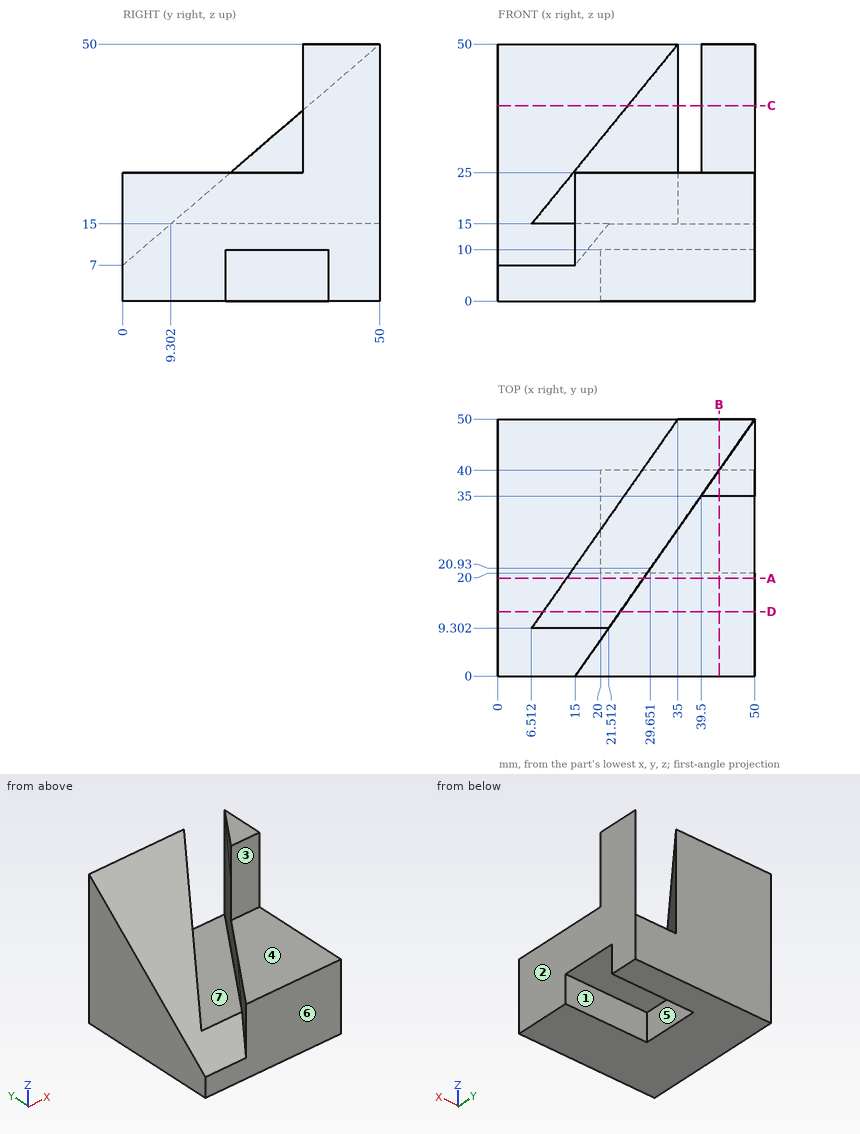
Can you work these out from the drawing? Everything is in mm from the part's minimum corner. A direction names the side the tool comes from. Coordinates: 2 decimals unless noted, no trailing zeros. Write each loop counter-clockwise with the first axis right and the second up, starting at its lowest first coordinate (ties: lowest second). Pieces come first, ordered by that corner, then holes. Notation, with made-up numbers: (-3.5, -21) -> (4.5, -21) arc R26 ccw to (4.5, 11) -> close; hole circle Ø9 at (67, 40). An arc over 180 degrees is marked (long way). Return JSON: item names as keys, results as strings.
(1) I'm going to push flat-ended pins straight in: pin 1 (8 mm diameter, centred on x = 5, y = 30.5, fed in from -Z); pin 2 (5 mm diameter, centred on x = 47, z = 37, fed in from -Y); pin 3 (3 mm diameter, centred on y = 28, z = 2.5, fed in from +X). Where does each tip first touch, or does it pass through?
Numbers:
{"pin 1": "stops at z = 0", "pin 2": "stops at y = 35", "pin 3": "stops at x = 20"}
(2) Imagine slicing it at A-A, the plane y = 19. Please give me the cut outline in (x, z).
Numbers:
{"outline": "(0, 0) -> (50, 0) -> (50, 25) -> (28.3, 25) -> (28.3, 15) -> (13.3, 15) -> (13.3, 23.34) -> (0, 23.34) -> close"}
(3) Imagine slicing it at B-B, the plane x = 43. Please give me the cut outline in (y, z).
Numbers:
{"outline": "(0, 0) -> (20, 0) -> (20, 10) -> (40, 10) -> (40, 0) -> (50, 0) -> (50, 15) -> (40, 15) -> (40, 50) -> (35, 50) -> (35, 25) -> (0, 25) -> close"}
(4) Which directions (+Z, -Z, +X, -X, +Y, -Y) give clear straight access to the entire face, cutting with the end or side of a thin tool? Please do the marked faces 1, 2 and 3.
Numbers:
{"face 1": "-Z, +X", "face 2": "+Z, -Z, +X, +Y, -Y", "face 3": "+Z, +X, -Y"}
(5) Imagine slicing it at D-D, the plane y = 12.5. Please give me the cut outline in (x, z), then the cut area to 3 significant figures.
Numbers:
{"outline": "(0, 0) -> (50, 0) -> (50, 25) -> (23.75, 25) -> (23.75, 15) -> (8.75, 15) -> (8.75, 17.75) -> (0, 17.75) -> close", "area": "1,040 mm2"}
(6) I need wall thicknesses on L1, parallel to Y at x = 34.5, z = 7; L2, parallel to Z at x = 29.5, y = 37; L3, parallel to Z at x = 41, y = 15. Which ranges of each line are inside material? Lowest first, please.
Numbers:
{"L1": "y = 0 to 20, 40 to 50", "L2": "z = 10 to 15", "L3": "z = 0 to 25"}
(7) We'd pull the mould along Y, two halves only. Please class the marked faces 4, 5, 6 and 7: +Y half, -Y half, draft (parallel to the pull), parting line (faces both ways), or undercut.
Numbers:
{"face 4": "draft", "face 5": "undercut", "face 6": "-Y half", "face 7": "undercut"}
(8) Imagine slicing it at C-C, the plane z = 38. Please give me the cut outline in (x, y).
Numbers:
{"outline": "(0, 36.05) -> (25.23, 36.05) -> (35, 50) -> (0, 50) -> close; (39.5, 35) -> (50, 35) -> (50, 50) -> close"}
